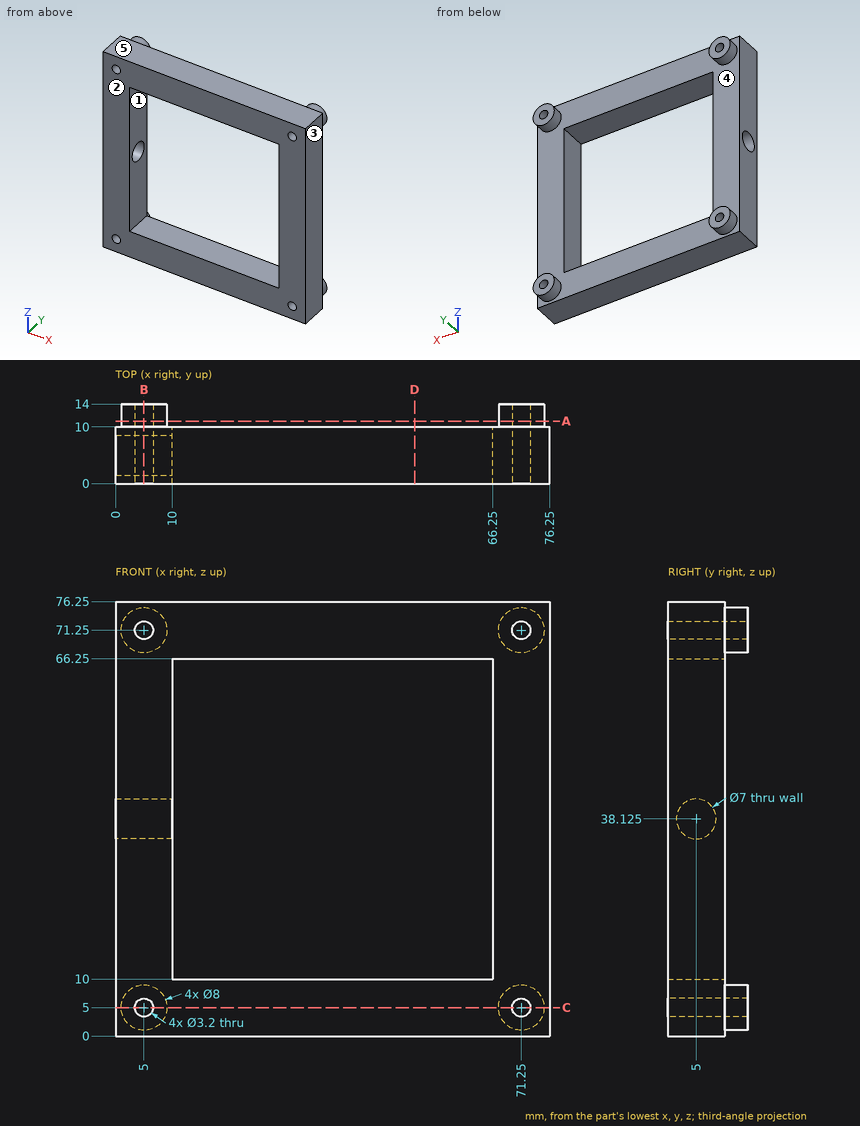
Input: dimensioned drawing with shaded views. Units: mm. Origin: part minimum x, y, z. A direction names the side the tool comes from. Coordinates: 2 decimals unless noted, no trailing zeros. Order: outer loops, then holes, each group sorted by start corner. A loop starts at its lowest first (then second) coordinate and runs counter-clockwise, first axis right, second up. Notation, with made-up numbers: (51.5, 25) -> (101.5, 25) arc R12 ccw to (101.5, 36) -> close; hole circle Ø6 at (41, -10). An arc over 180 degrees is marked (long way). Answer in a Markdown table with one row per item.
Item 1: Ray query, L1, parallel to X at y = 10.5, z = 5; L2, parallel to X at y = 6, z = 5. Return the intervals inside material, ascending.
Return value:
| item | result |
|---|---|
| L1 | x = 1 to 3.4, 6.6 to 9, 67.25 to 69.65, 72.85 to 75.25 |
| L2 | x = 0 to 3.4, 6.6 to 69.65, 72.85 to 76.25 |
Item 2: Access query for the marked faces 1 and 2. Directions: +Z, -Z, +X, -X, +Y, -Y. A direction counts if a zero-diameter tool reaches every point of the face in a straight line with its end or side. Return the directions, or none.
Return value:
| item | result |
|---|---|
| face 1 | +Y, -Y |
| face 2 | +Z, -Z, +X, -X, -Y |
Item 3: Section C-C on z = 5. Output: boundary loops of the cut face in (x, y), plus the area to 3 significant figures.
Return value:
| item | result |
|---|---|
| outline | (0, 0) -> (3.4, 0) -> (3.4, 14) -> (1, 14) -> (1, 10) -> (0, 10) -> close; (6.6, 0) -> (69.65, 0) -> (69.65, 14) -> (67.25, 14) -> (67.25, 10) -> (9, 10) -> (9, 14) -> (6.6, 14) -> close; (72.85, 0) -> (76.25, 0) -> (76.25, 10) -> (75.25, 10) -> (75.25, 14) -> (72.85, 14) -> close |
| area | 737 mm² |
Item 4: Contact query for a flat-ended pin moving along its axis: P1, Ø3, axis at y = 6, z = 38, coming from the -X side. Output: stop coordinate, or through.
Return value:
| item | result |
|---|---|
| P1 | stops at x = 66.25 |
Item 5: Section A-A on y = 11. Output: boundary loops of the cut face in (x, z).
Return value:
| item | result |
|---|---|
| outline | circle Ø8 at (5, 5); circle Ø8 at (5, 71.25); circle Ø8 at (71.25, 5); circle Ø8 at (71.25, 71.25); hole circle Ø3.2 at (5, 5); hole circle Ø3.2 at (5, 71.25); hole circle Ø3.2 at (71.25, 5); hole circle Ø3.2 at (71.25, 71.25) |
Item 6: Section B-B on x = 5. Output: boundary loops of the cut face in (y, z) (3 decimals), plus the area to 3 significant figures.
Return value:
| item | result |
|---|---|
| outline | (0, 0) -> (10, 0) -> (10, 1) -> (14, 1) -> (14, 3.4) -> (0, 3.4) -> close; (0, 6.6) -> (14, 6.6) -> (14, 9) -> (10, 9) -> (10, 67.25) -> (14, 67.25) -> (14, 69.65) -> (0, 69.65) -> close; (0, 72.85) -> (14, 72.85) -> (14, 75.25) -> (10, 75.25) -> (10, 76.25) -> (0, 76.25) -> close; hole circle Ø7 at (5, 38.125) |
| area | 698 mm² |
Item 7: Section D-D on x = 52.5. Output: boundary loops of the cut face in (y, z).
Return value:
| item | result |
|---|---|
| outline | (0, 0) -> (10, 0) -> (10, 10) -> (0, 10) -> close; (0, 66.25) -> (10, 66.25) -> (10, 76.25) -> (0, 76.25) -> close |
Item 8: Draft query along X for the marked faces 3, 4 and 5. Return one class per face: released by +X, released by -X, zero draft, split by the parting line, or undercut.
Return value:
| item | result |
|---|---|
| face 3 | released by +X |
| face 4 | undercut |
| face 5 | zero draft |
